Source: CAD feature listing. Evaluate the final solid. Frame: model axes, mm. A direction names the side the tool comes from. Coordinates: 2 decimals unless noted, no trailing zeros. Loops run counter-clockwise (first coordinate to the right, second up) from the corner with the lowest first, then second, coordinate; pieces in that order, holes last.
from build123d import *

# Parameters (mm, degrees)
F0_W     = 87.9665389657
F0_H     = 87.1540307999
F1_DEPTH = 44
F2_W     = 74.8088378459
F2_H     = 74.356541276
F3_DEPTH = 72
F4_W     = 74.356541276
F4_H     = 25.3268238157
F5_DEPTH = 13.1587011198
F6_R     = 20


with BuildPart() as f1:
    # F0 (on Front) → F1 (new body, symmetric)
    with BuildSketch(Plane.XZ):
        Rectangle(F0_W, F0_H)
    extrude(amount=F1_DEPTH, both=True)

    # F2 (on face) → F3 (cut)
    with BuildSketch(Plane.XY.offset(43.5770153999)):
        with Locations((6.5788505599, -6.821729362)):
            Rectangle(F2_W, F2_H)
    extrude(amount=-F3_DEPTH, mode=Mode.SUBTRACT)

    # F4 (on face) → F5 (cut, through all)
    with BuildSketch(Plane.YZ.offset(-30.8255683631)):
        with Locations((-6.821729362, 30.9136034921)):
            Rectangle(F4_W, F4_H)
    extrude(amount=-F5_DEPTH, mode=Mode.SUBTRACT)

    # F6
    f6_edges = [f1.edges().sort_by_distance(p)[0] for p in [
        (43.983269, 37.178271, 43.577015),
        (-37.404419, -44, 18.250192),
    ]]
    fillet(f6_edges, radius=F6_R)


solid = f1.part
Q1. Section A-A, the plane x = -27. Return the cut outline in (y, z), plus the area to 3 significant figures.
Q2. Section B-B, the plane y = 10. Return the cut outline in (x, z).
Q3. Contact query for flat-ended pins moving along their axis: pin 1 Ø1 at (y, z) = (-19.5, -2) entering from +X; pin 2 Ø6.5 at (x, y) = (-35.5, -5.5) entering from +Z; pin 3 Ø3 at (x, z) = (12, -17.5) entering from -Y. Output: stop coordinate, or through.
Q4. Section C-C, the plane z = 30. Return the cut outline in (x, y), plus the area to 3 significant figures.
Q5. Line query: line 1 along X through (y, z) = (-14.5, -8); line 2 along Y through (x, z) = (14.5, 29); line 3 along Z through (x, y) = (21.5, -22). Output: solid intervals per line, ascending.
Q6. Access query for faces 1 (the flat face through (-10, -44, -32)), 2 (the flat face through (-30.826, -7, -5)), 3 (the flat face through (-37, 3, 18.25)). Directions: +Z, -Z, +X, -X, +Y, -Y. A direction counts if a zero-diameter tool reaches every point of the face in a straight line with its end or side. Return the directions, or none.
Derived:
1. outline: (-44, -43.58) - (44, -43.58) - (44, 43.58) - (30.36, 43.58) - (30.36, -28.42) - (-44, -28.42) - close
1. area: 2,320 mm2
2. outline: (-43.98, -43.58) - (43.98, -43.58) - (43.98, -28.42) - (-30.83, -28.42) - (-30.83, 18.25) - (-43.98, 18.25) - close
3. pin 1: stops at x = -30.83
3. pin 2: stops at z = 18.25
3. pin 3: stops at y = 30.36
4. outline: (-43.98, 30.36) - (42.92, 30.36) - (42.92, 44) - (-43.98, 44) - close
4. area: 1,190 mm2
5. line 1: x = -43.98 to -30.83
5. line 2: y = 30.36 to 44
5. line 3: z = -43.58 to -28.42
6. face 1: +Z, -Z, +X, -X, -Y
6. face 2: +Z, +X, -Y
6. face 3: +Z, +X, -X, -Y
